For this review, take the finished solid that the model builds, in its own axes (mm). Face numbers are marked on the shaded views. Give positions to 0.01 mm unless a question says otherwise; leave off trailing zeros. Order: outer loops, then holes, each group sorted by start corner. A loop starts at its lowest first (then second) coordinate and runs counter-clockwise, first axis right, second up. Notation, with made-up numbers: (-22.75, 41.5) - (5.25, 41.5) arc R35 cw to (5.25, 75.5) - close; hole circle Ø4 at (31.25, -1). An arc over 180 degrees is marked (long way). Use a Markdown table: item, result. Add a question column.
1) Clearance check with flat-ended pins moving along their axes: P1, Ø2, axis at x = 1, y = -6, coming from the +Z side; P2, Ø1, axis at x = -1.5, z = 6.5, coming from the -Y side; P3, Ø1, axis at x = 2.5, z = 2, coming from the -Y side. State where each tip first meets the part, or that it passes through.
2) We need section C-C on z = 5.25. Write out the cut boundary in (x, y).
3) Wall thickness on L1, parallel to Y at x = 0, z = 4.5; L2, parallel to Z at x = 3.75, y = 1.25; L3, parallel to X at y = 3.75, z = 5.75: over which ranges is each line inside the solid? List them lowest first.
4) We need section A-A on x = 0. Write out the cut boundary in (y, z).
5) Mouldability with a two-part tool opening along Y and no side actions: class the marked faces 1, 2 and 3 as released by +Y, released by -Y, zero draft, split by the parting line, or undercut.
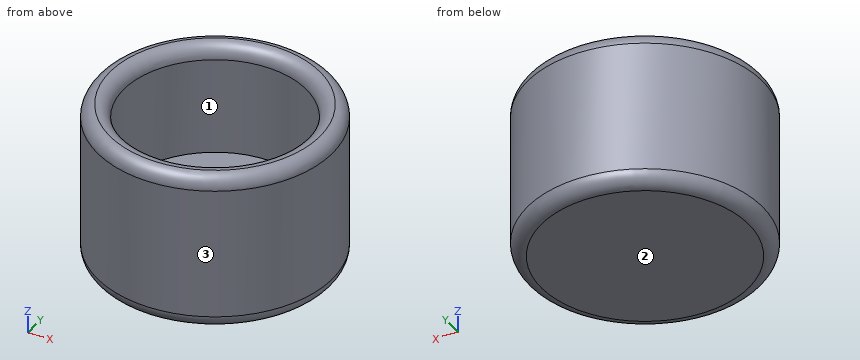
```python
from build123d import *

# Parameters (mm, degrees)
F0_R     = 8.5
F1_DEPTH = 3.5
F2_R     = 8.5
F2_R_2   = 6.6
F3_DEPTH = 8
F4_R     = 1


# Not quite as in the source:
# - a fillet or chamfer that OpenCascade refuses, or shapes differently, is made with other operations: its cross-section is extruded or revolved along the edge and cut away or added
# - a feature names something its author has since deleted; it is built from what else it names


with BuildPart() as f1:
    # F0 (on Top) → F1 (new body)
    with BuildSketch(Plane.XY):
        Circle(F0_R)
    extrude(amount=-F1_DEPTH)

    # F2 (on face) → F3 (join)
    with BuildSketch(Plane.XY):
        Circle(F2_R)
        Circle(F2_R_2, mode=Mode.SUBTRACT)
    extrude(amount=F3_DEPTH)

    # F4
    f4_edges = [f1.edges().sort_by_distance(p)[0] for p in [
        (-6.6, 0, 8),
        (-8.5, 0, -3.5),
    ]]
    fillet(f4_edges, radius=F4_R)

    # F5: fillet of radius 1 on 1 edges, made by hand

    # F5_s1 → F5_t2 (revolve, cut)
    with BuildSketch(Plane.XZ):
        with BuildLine():
            ThreePointArc((8.5, 7.0050125629), (8.2416198487, 7.6758329561), (7.6, 8))
            Line((7.6, 8), (8.5, 8))
            Line((8.5, 8), (8.5, 7.0050125629))
        make_face()
    revolve(axis=Axis((0, 0, 8), (0, 0, 1)), mode=Mode.SUBTRACT)


solid = f1.part
```
Checked values:
| question | item | result |
|---|---|---|
| 1 | P1 | z = 7.86 |
| 1 | P2 | y = -8.44 |
| 1 | P3 | y = -8.26 |
| 2 | outline | circle Ø17 at (0, 0); hole circle Ø13.2 at (0, 0) |
| 3 | L1 | -8.5 to -6.6, 6.6 to 8.5 |
| 3 | L2 | -3.5 to 0 |
| 3 | L3 | -7.63 to -5.43, 5.43 to 7.63 |
| 4 | outline | (-8.5, -2.5) arc R1 ccw to (-7.5, -3.5) - (7.5, -3.5) arc R1 ccw to (8.5, -2.5) - (8.5, 7.01) arc R1 ccw to (7.6, 8) arc R1 ccw to (6.6, 7) - (6.6, 0) - (-6.6, 0) - (-6.6, 7) arc R1 ccw to (-7.6, 8) arc R1 ccw to (-8.5, 7.01) - close |
| 5 | face 1 | undercut |
| 5 | face 2 | zero draft |
| 5 | face 3 | split by the parting line |
